```python
from build123d import *

# Parameters (mm, degrees)
EXTRUDE_THIN1_DEPTH = 17
FILLET1_R           = 2
FILLET2_R           = 2
SKETCH2_R           = 2.25
CUT_EXTRUDE1_DEPTH  = 10
SKETCH4_R           = 2.25
CUT_EXTRUDE2_DEPTH  = 10


with BuildPart() as part:
    # Sketch1 → Extrude-Thin1 (new body)
    with BuildSketch(Plane.XY):
        Polygon((0, 30), (0, 0), (30, 0), (30, 2), (2, 2), (2, 30), align=None)
    extrude(amount=EXTRUDE_THIN1_DEPTH)

    # Fillet1
    fillet1_edges = [part.edges().sort_by_distance(p)[0] for p in [
        (1, 30, 17),
        (1, 30, 0),
        (30, 1, 0),
        (30, 1, 17),
    ]]
    fillet(fillet1_edges, radius=FILLET1_R)

    # Fillet2
    fillet2_edges = [part.edges().sort_by_distance(p)[0] for p in [
        (0, 0, 8.5),
        (2, 2, 8.5),
    ]]
    fillet(fillet2_edges, radius=FILLET2_R)

    # Sketch2 → Cut-Extrude1 (cut)
    with BuildSketch(Plane.ZY):
        with Locations((8.5, 20)):
            Circle(SKETCH2_R)
    extrude(amount=-CUT_EXTRUDE1_DEPTH, mode=Mode.SUBTRACT)

    # Sketch4 → Cut-Extrude2 (cut)
    with BuildSketch(Plane.XZ):
        with Locations(Location((20, 8.5, 0), (0, 0, 270))):
            Circle(SKETCH4_R)
    extrude(amount=-CUT_EXTRUDE2_DEPTH, mode=Mode.SUBTRACT)


solid = part.part
```
The listing builds one solid part. Answer for the finished solid, in the listing's coordinates (mm). A direction names the side the tool comes from. Give positions to 0.01 mm unless a question says otherwise; leave off trailing zeros. Write each loop counter-clockwise with the first axis right and the second up, starting at its lowest first coordinate (ties: lowest second). Pieces come first, ordered by that corner, then holes. Notation, with made-up numbers: (-33, 48) -> (2, 48) arc R27 ccw to (2, 67) -> close; hole circle Ø5 at (73, 84). An arc over 180 degrees is marked (long way). Write item = value, one per line. Start each with the question number.
1) The part is cut by section C-C, the plane z = 8.5. Determine the outline of the cut face in (x, y), and give its area (3 significant figures).
2) Determine the mould class of faces 3 (the face through (30, 1, 8)), 4 (the face through (1, 8, 0)), 5 (the face through (17.804, 0.986, 8.988)) for opening direction X: +X half, -X half, draft (parallel to the pull), parting line (faces both ways), or undercut.
3) The part is cut by section A-A, the plane x = 20. Determine the outline of the cut face in (y, z).
4) Straight lines are drawn through the part: line 1 along X through (y, z) = (12.5, 12.5); line 2 along X through (y, z) = (1.15, 8.5). For each, find the intervals that lie inside material, in ascending order.
5) The part is cut by section D-D, the plane z = 3. Determine the outline of the cut face in (x, y).
6) This flat-tipped pin is pushed along its axis until it touches: pin 1 (6 mm diameter, centred on x = 20, z = 8.5, fed in from +Y). Where does it stop, or does it pass through?
7) Which of the six approach directions +Z, -Z, +X, -X, +Y, -Y give full straight-line access (tool end or side, diameter ignored) to faces 1 (the face through (29.43, 1.01, 16.4)), 2 (the face through (17, 2, 8))?
Solutions:
q1.outline = (0, 2) arc R2 ccw to (2, 0) -> (17.75, 0) -> (17.75, 2) -> (4, 2) arc R2 cw to (2, 4) -> (2, 17.75) -> (0, 17.75) -> close; (0, 22.25) -> (2, 22.25) -> (2, 30) -> (0, 30) -> close; (22.25, 0) -> (30, 0) -> (30, 2) -> (22.25, 2) -> close
q1.area = 98.0 mm²
q2.face_3 = +X half
q2.face_4 = draft
q2.face_5 = undercut
q3.outline = (0, 0) -> (2, 0) -> (2, 6.25) -> (0, 6.25) -> close; (0, 10.75) -> (2, 10.75) -> (2, 17) -> (0, 17) -> close
q4.line_1 = 0 to 2
q4.line_2 = 0.19 to 17.75, 22.25 to 30
q5.outline = (0, 2) arc R2 ccw to (2, 0) -> (30, 0) -> (30, 2) -> (4, 2) arc R2 cw to (2, 4) -> (2, 30) -> (0, 30) -> close
q6.pin_1 = 2
q7.face_1 = +Z, +X, +Y, -Y
q7.face_2 = +Z, -Z, +X, +Y
